from build123d import *

# Parameters (mm, degrees)
F1_DEPTH = 5
F2_R     = 50.8
F3_R     = 14.224
F5_D     = 4.4


with BuildPart() as f1:
    # F0 (on Top) → F1 (new body)
    with BuildSketch(Plane.XY):
        Polygon((0, 100), (-100, 0), (100, 0), align=None)
    extrude(amount=F1_DEPTH)

    # F2
    f2_edges = [f1.edges().sort_by_distance(p)[0] for p in [
        (0, 100, 2.5),
    ]]
    fillet(f2_edges, radius=F2_R)

    # F3
    f3_edges = [f1.edges().sort_by_distance(p)[0] for p in [
        (-100, 0, 2.5),
        (100, 0, 2.5),
    ]]
    fillet(f3_edges, radius=F3_R)

    # F5 (through all)
    with Locations(Plane.XY.offset(5)):
        with Locations((-28.8579897851, 58.5696516454), (28.8579897851, 58.5696516454), (60.2944809943, 8.89), (-60.2944809943, 8.89)):
            Hole(F5_D / 2)


solid = f1.part
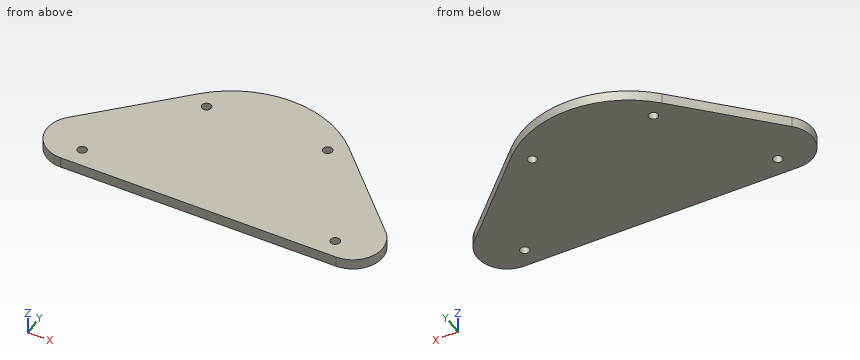
Model file for the job. Use its own axes, mm. Give positions to 0.01 mm unless a question says otherwise; leave off trailing zeros. Loops run counter-clockwise (first coordinate to the right, second up) from the corner with the lowest first, then second, coordinate; pieces in that order, holes last.
Item 1: Drop flat-ended pins along their axis: P1, Ø2.5, axis at x = -60.29, y = 8.89, coming from the +Z side; P2, Ø1.5, axis at x = -51.5, z = 1.5, coming from the +Y side; P3, Ø1.5, axis at y = 35.5, z = 3, coming from the -X side; P4, Ø3, axis at x = 62, z = 4, coming from the +Y side. Give the stop position or say it passes through.
Check values:
P1: passes through
P2: stops at y = 49.25
P3: stops at x = -65.25
P4: stops at y = 39.5
Item 2: Drill centre lines: line 1 along Y through (x, z) = (28, 0.85); line 2 along Y through (x, z) = (60.5, 3.6); line 3 along Y through (x, z) = (69, 2.7). Where is each one in solid material? Low to high.
Check values:
line 1: y = 0 to 56.54, 60.6 to 70.54
line 2: y = 0 to 6.7, 11.08 to 39.5
line 3: y = 0.4 to 31
Item 3: Slice it at D-D (y = 27). Write the cut outline in (x, z).
Check values:
outline: (-73, 0) - (73, 0) - (73, 5) - (-73, 5) - close
Item 4: Slice it at A-A (y = 8.89). Write the cut outline in (x, z).
Check values:
outline: (-78.85, 0) - (-62.49, 0) - (-62.49, 5) - (-78.85, 5) - close; (-58.09, 0) - (58.09, 0) - (58.09, 5) - (-58.09, 5) - close; (62.49, 0) - (78.85, 0) - (78.85, 5) - (62.49, 5) - close
Item 5: Slice it at C-C (z = 3.45). Write the cut outline in (x, y), plus the area to 3 significant figures.
Check values:
outline: (-75.72, 24.28) arc R14.22 ccw to (-65.66, 0) - (65.66, 0) arc R14.22 ccw to (75.72, 24.28) - (35.92, 64.08) arc R50.8 ccw to (-35.92, 64.08) - close; hole circle Ø4.4 at (-60.29, 8.89); hole circle Ø4.4 at (-28.86, 58.57); hole circle Ø4.4 at (28.86, 58.57); hole circle Ø4.4 at (60.29, 8.89)
area: 8,890 mm2
Item 6: Slice it at B-B (x = 60). Write the cut outline in (y, z), plus the area to 3 significant figures.
Check values:
outline: (0, 0) - (6.71, 0) - (6.71, 5) - (0, 5) - close; (11.07, 0) - (40, 0) - (40, 5) - (11.07, 5) - close
area: 178 mm2
